```python
from build123d import *

# Parameters (mm, degrees)
SKETCH_1_W               = 14.3
SKETCH_1_H               = 14.3
SKETCH_1_W_2             = 10.3
SKETCH_1_H_2             = 10.3
EXTRUDE_1_DEPTH          = 35
EXTRUDE_1_2_DEPTH        = 14.3
CUT_EXTRUDE_1_DEPTH      = 52.538771813
CUT_EXTRUDE_1_DEPTH_BACK = 52.538771813
SKETCH_3_R               = 1.65
SKETCH_3_4_R             = 1.65
CUT_EXTRUDE_2_DEPTH      = 52.538771813
CUT_EXTRUDE_START        = -14.3
SKETCH_3_5_R             = 1.65
CUT_EXTRUDE_3_DEPTH      = 38.238771813
CUT_EXTRUDE_4_REACH      = 48.649
SKETCH_4_R               = 2.65
CUT_EXTRUDE_START_2      = -13.129103
SKETCH_4_3_R             = 5
CUT_EXTRUDE_5_DEPTH      = 7.129103
CHAMFER_1_SIZE           = 1


with BuildPart() as part:
    # 草图1 → Extrude 1 (new body)
    with BuildSketch(Plane.XY):
        Rectangle(SKETCH_1_W, SKETCH_1_H)
        Rectangle(SKETCH_1_W_2, SKETCH_1_H_2, mode=Mode.SUBTRACT)
    extrude(amount=EXTRUDE_1_DEPTH)

    # 草图2 → Extrude 1 2 (add)
    with BuildSketch(Plane.ZY.offset(7.15)):
        Polygon((0, 30), (0, 7.15), (20, 7.15), align=None)
        Polygon((0, -7.15), (0, -30), (20, -7.15), align=None)
    extrude(amount=-EXTRUDE_1_2_DEPTH)

    # 草图3 → 切除-拉伸1 (cut, two sides: drawn at the far end of the back side and taken through both)
    with BuildSketch(Plane.XZ.offset(7.15).offset(-CUT_EXTRUDE_1_DEPTH_BACK)):
        with Locations((0, 30)):
            Circle(SKETCH_3_R)
        with Locations(Location((0, 17.5, 0), (0, 0, 270))):
            Circle(SKETCH_3_R)
    extrude(amount=CUT_EXTRUDE_1_DEPTH + CUT_EXTRUDE_1_DEPTH_BACK, mode=Mode.SUBTRACT)

    # 草图3<4> → 切除-拉伸2 (cut, through all)
    # profile 1 of 2: a face of its own
    with BuildSketch(Plane.XZ.offset(7.15)):
        with BuildLine():
            ThreePointArc((-3.122498999, 20), (-1.324764885, 13.725745372), (4, 17.5))
            ThreePointArc((4, 17.5), (3.774254628, 18.824764885), (3.122498999, 20))
            Line((3.122498999, 20), (-3.122498999, 20))
        make_face()
        with Locations((0, 17.5)):
            Circle(SKETCH_3_4_R, mode=Mode.SUBTRACT)
    # profile 2 of 2: a face of its own
    with BuildSketch(Plane.XZ.offset(7.15)):
        with BuildLine():
            ThreePointArc((-3.122498999, 20), (-1.324764885, 13.725745372), (4, 17.5))
            ThreePointArc((4, 17.5), (3.774254628, 18.824764885), (3.122498999, 20))
            Line((3.122498999, 20), (-3.122498999, 20))
        make_face()
        with Locations((0, 17.5)):
            Circle(SKETCH_3_4_R, mode=Mode.SUBTRACT)
    extrude(amount=CUT_EXTRUDE_2_DEPTH, mode=Mode.SUBTRACT)

    # 草图3<5> → 切除-拉伸3 (cut, through all)
    # profile 1 of 2: a face of its own
    with BuildSketch(Plane.XZ.offset(7.15).offset(CUT_EXTRUDE_START)):
        with BuildLine():
            ThreePointArc((-3.122498999, 20), (-1.324764885, 13.725745372), (4, 17.5))
            ThreePointArc((4, 17.5), (3.774254628, 18.824764885), (3.122498999, 20))
            Line((3.122498999, 20), (-3.122498999, 20))
        make_face()
        with Locations((0, 17.5)):
            Circle(SKETCH_3_5_R, mode=Mode.SUBTRACT)
    # profile 2 of 2: a face of its own
    with BuildSketch(Plane.XZ.offset(7.15).offset(CUT_EXTRUDE_START)):
        with BuildLine():
            ThreePointArc((-3.122498999, 20), (-1.324764885, 13.725745372), (4, 17.5))
            ThreePointArc((4, 17.5), (3.774254628, 18.824764885), (3.122498999, 20))
            Line((3.122498999, 20), (-3.122498999, 20))
        make_face()
        with Locations((0, 17.5)):
            Circle(SKETCH_3_5_R, mode=Mode.SUBTRACT)
    extrude(amount=-CUT_EXTRUDE_3_DEPTH, mode=Mode.SUBTRACT)

    # 草图4 → 切除-拉伸4 (cut, up to next)
    with BuildSketch(Plane(origin=(0, 0, 0), x_dir=(-1, 0, 0), z_dir=(0, 0, -1)), mode=Mode.PRIVATE) as cut_extrude_4_sk1:
        with Locations((0, 20)):
            Circle(SKETCH_4_R)
    cut_extrude_4_tool1 = extrude(cut_extrude_4_sk1.sketch, amount=-CUT_EXTRUDE_4_REACH, mode=Mode.PRIVATE) & part.part
    # 草图4 → 切除-拉伸4 (cut, up to next)
    with BuildSketch(Plane(origin=(0, 0, 0), x_dir=(-1, 0, 0), z_dir=(0, 0, -1)), mode=Mode.PRIVATE) as cut_extrude_4_sk2:
        with Locations((0, -20)):
            Circle(SKETCH_4_R)
    cut_extrude_4_tool2 = extrude(cut_extrude_4_sk2.sketch, amount=-CUT_EXTRUDE_4_REACH, mode=Mode.PRIVATE) & part.part
    add(cut_extrude_4_tool1.solids().sort_by_distance((0, 20, 0))[0], mode=Mode.SUBTRACT)
    add(cut_extrude_4_tool2.solids().sort_by_distance((0, -20, 0))[0], mode=Mode.SUBTRACT)

    # 草图4<3> → 切除-拉伸5 (cut)
    with BuildSketch(Plane(origin=(0, 0, 0), x_dir=(-1, 0, 0), z_dir=(0, 0, -1)).offset(CUT_EXTRUDE_START_2)):
        with Locations((0, 20)):
            Circle(SKETCH_4_3_R)
        with Locations((0, -20)):
            Circle(SKETCH_4_3_R)
    extrude(amount=CUT_EXTRUDE_5_DEPTH, mode=Mode.SUBTRACT)

    # 倒角1
    chamfer_1_edges = [part.edges().sort_by_distance(p)[0] for p in [
        (7.15, 0, 35),
        (0, 7.15, 35),
        (-7.15, 0, 35),
        (0, -7.15, 35),
    ]]
    chamfer(chamfer_1_edges, length=CHAMFER_1_SIZE)


solid = part.part
```
Geometry check sheet. Reference: the model listing, model coordinates, mm. A direction names the side the tool comes from. Give positions to 0.01 mm unless a question says otherwise; leave off trailing zeros. Order: outer loops, then holes, each group sorted by start corner. A loop starts at its lowest first (then second) coordinate and runs counter-clockwise, first axis right, second up.
1. Thickness scan on L1, parallel to Z at x = 0, y = -5.55; L2, parallel to X at y = 2, z = 8; L3, parallel to Y at x = 0, z = 9.75. Record the ranges inside material, lowest first.
2. Release check for a two-part mould opening along X. For faces 4 (the face through (0, 7.15, 26)), 5 (the face through (7.15, 0, 13)), 6 (the face through (-7.15, 0, 13)), 7 (the face through (-6, 0, 0)) record: pulls with the +X half, pulls with the -X half, needs draft (parallel to the pull), parting line crosses it, or undercut.
3. Access from +Z, -Z, +X, -X, +Y, -Y to the whole of each face (thin tool, end or side, straight path). Record for faces 1 (the face through (0.07, -6.14, 19.15)), 2 (the face through (0, -17, 6)), 3 (the face through (-5.15, 0, 17)).
4. Section check C-C, the plane z = 30. Enter the section's corners in (x, y), and give its area (3 significant figures).
5. Gauge pin test, flat ends, axial feed: pin 1 Ø8 at (x, y) = (-3, 10.5) entering from +Z; pin 2 Ø2 at (x, z) = (0, 30) entering from -Y; pin 3 Ø7 at (x, z) = (2.5, 24.5) entering from -Y; pin 4 Ø6 at (x, z) = (-4, 22.5) entering from -Y. Record the tip position at first contact, or that the pin passes through.
6. Section check D-D, the plane x = 0. Give the number of separate pieces and of enclosed holes in the cut face, and give its area (3 significant figures).
7. Section check A-A, the plane z = 24.5. Enter the section's corners in (x, y).
8. Section check B-B, the plane y = 3.5. Enter the section's corners in (x, z), and give its area (3 significant figures).
Values follow:
1. L1: z = 0 to 15.85, 19.15 to 28.35, 31.65 to 35
1. L2: x = -7.15 to -5.15, 5.15 to 7.15
1. L3: y = -15 to -5.15, 5.15 to 15
2. face 4: undercut
2. face 5: pulls with the +X half
2. face 6: pulls with the -X half
2. face 7: needs draft
3. face 1: +Y, -Y
3. face 2: +Z
3. face 3: +Z, -Z
4. outline: (-7.15, -7.15) - (-1.65, -7.15) - (-1.65, -5.15) - (-5.15, -5.15) - (-5.15, 5.15) - (-1.65, 5.15) - (-1.65, 7.15) - (-7.15, 7.15) - close; (1.65, -7.15) - (7.15, -7.15) - (7.15, 7.15) - (1.65, 7.15) - (1.65, 5.15) - (5.15, 5.15) - (5.15, -5.15) - (1.65, -5.15) - close
4. area: 85.2 mm2
5. pin 1: stops at z = 34.65
5. pin 2: passes through
5. pin 3: stops at y = -7.15
5. pin 4: stops at y = -7.72
6. separate pieces: 8
6. enclosed holes: 0
6. area: 400 mm2
7. outline: (-7.15, -7.15) - (7.15, -7.15) - (7.15, 7.15) - (-7.15, 7.15) - close; hole (-5.15, -5.15) - (5.15, -5.15) - (5.15, 5.15) - (-5.15, 5.15) - close
8. outline: (-7.15, 0) - (-5.15, 0) - (-5.15, 35) - (-6.15, 35) - (-7.15, 34) - close; (5.15, 0) - (7.15, 0) - (7.15, 34) - (6.15, 35) - (5.15, 35) - close
8. area: 139 mm2
